Verification items for the finished model (mm, model axes). Round coordinates to 2 decimals unless told otherwise and drop trailing zeros. Order: outer loops, then holes, each group sorted by start corner. A loop starts at its lowest first (then second) coordinate and runs counter-clockwise, first axis right, second up.
```python
from build123d import *

# Parameters (mm, degrees)
F1_DEPTH = 1800
F2_R     = 0.5
F3_R     = 1.5
F4_R     = 2.1
F5_DEPTH = 25


with BuildPart() as f1:
    # F0 (on Right) → F1 (new body)
    with BuildSketch(Plane.YZ):
        Polygon((-12, 0), (0, 0), (0, 10), (-1, 10), (-1, 1), (-12, 1), align=None)
    extrude(amount=F1_DEPTH)

    # F2
    f2_edges = [f1.edges().sort_by_distance(p)[0] for p in [
        (900, -1, 1),
    ]]
    fillet(f2_edges, radius=F2_R)

    # F3
    f3_edges = [f1.edges().sort_by_distance(p)[0] for p in [
        (900, 0, 0),
    ]]
    fillet(f3_edges, radius=F3_R)

    # F4 (on Top) → F5 (cut)
    with BuildSketch(Plane.XY):
        with Locations((30, -6.5)):
            Circle(F4_R)
        with Locations((378, -6.5)):
            Circle(F4_R)
        with Locations((726, -6.5)):
            Circle(F4_R)
        with Locations((1074, -6.5)):
            Circle(F4_R)
        with Locations((1422, -6.5)):
            Circle(F4_R)
        with Locations((1770, -6.5)):
            Circle(F4_R)
    extrude(amount=F5_DEPTH, mode=Mode.SUBTRACT)


solid = f1.part
```
1) Sectioned sample at B-B on x = 1358. Record the cut outline in (y, z), then the cut area to 3 significant figures.
2) Sectioned sample at A-A on y = -6.5. Record the cut outline in (x, z), then the cut area to 3 significant figures.
3) Sectioned sample at C-C on z = 3. Record the cut outline in (x, y).
4) Scan lines: probe 1 along Y at (x, z) = (1074, 0.75); probe 2 along Z at (x, y) = (647.5, -4.75); probe 3 along Y at (x, z) = (167.5, 9.25). Record each from-to range of solid material in increasing order.
5) Go/stop test with flat-tipped pins: pin 1 Ø4 at (x, y) = (1494.5, -8) entering from +Z; pin 2 Ø2.5 at (x, z) = (1093.5, 6.5) entering from -Y. Record where each tip stops, or that it passes through.
Returned:
1. outline: (-12, 0) - (-1.5, 0) arc R1.5 ccw to (0, 1.5) - (0, 10) - (-1, 10) - (-1, 1.5) arc R0.5 cw to (-1.5, 1) - (-12, 1) - close
1. area: 20.6 mm2
2. outline: (0, 0) - (27.9, 0) - (27.9, 1) - (0, 1) - close; (32.1, 0) - (375.9, 0) - (375.9, 1) - (32.1, 1) - close; (380.1, 0) - (723.9, 0) - (723.9, 1) - (380.1, 1) - close; (728.1, 0) - (1071.9, 0) - (1071.9, 1) - (728.1, 1) - close; (1076.1, 0) - (1419.9, 0) - (1419.9, 1) - (1076.1, 1) - close; (1424.1, 0) - (1767.9, 0) - (1767.9, 1) - (1424.1, 1) - close; (1772.1, 0) - (1800, 0) - (1800, 1) - (1772.1, 1) - close
2. area: 1,770 mm2
3. outline: (0, -1) - (1800, -1) - (1800, 0) - (0, 0) - close
4. probe 1: y = -12 to -8.6, -4.4 to -0.2
4. probe 2: z = 0 to 1
4. probe 3: y = -1 to 0
5. pin 1: stops at z = 1
5. pin 2: stops at y = -1
